Can you work these out from the model? Positions are in its coordinate system, mm. Face numbers are marked on the shaded views. Round coordinates to 2 decimals unless told otherwise and drop trailing zeros. Order: outer loops, then holes, each group sorted by start corner. A loop starts at its lowest first (then second) coordinate and runs counter-clockwise, first axis right, second up.
Q1. If we section it at B-B (y = 35): Please give me the cut outline in (x, z).
Q2. If I drill on line 1 (Z direction, x = 2, y = 7); line 2 (Z direction, x = 32, y = 17); line 3 (X direction, y = 4.5, z = -5), over which ranges is the centre line in solid material (lowest first)?
Q3. Will these pins go through, and if not, where does the flat tip stop? P1, Ø3, axis at x = 28.5, z = -0.5, coming from the +Y side; P2, Ø1.5, axis at y = 42, z = 2, coming from the -X side; P3, Ø3, axis at x = 75.5, y = 16, coming from the -Z side; P4, Ø1.1, axis at y = 8.5, z = 4, coming from the -X side.
Q4. If we section it at C-C (x = 2): Please give me the cut outline in (y, z), plus the area to 3 significant figures.
Q5. We'd pull the mould along Z, two halves only. Please class the marked faces 1, 2 and 3: pulls with the +Z half, pulls with the -Z half, needs draft (parallel to the pull), parting line crosses it, or undercut.
Q6. If we section it at A-A (z = -5): Please give me the cut outline in (x, y), plus the area to 3 significant figures.
Q7. If we section it at D-D (x = 46): Please give me the cut outline in (y, z).
from build123d import *

# Parameters (mm, degrees)
SKETCH1_R               = 5.501178274
BOSS_EXTRUDE1_DEPTH     = 5
SKETCH2_R               = 8
SKETCH2_R_2             = 5
BOSS_EXTRUDE2_DEPTH     = 70
CUT_EXTRUDE1_DEPTH      = 123.755855257
CUT_EXTRUDE1_DEPTH_BACK = 123.755855257
SKETCH3_W               = 17.823798536
SKETCH3_H               = 40


with BuildPart() as part:
    # Sketch1 → Boss-Extrude1 (new body)
    with BuildSketch(Plane.XY):
        Polygon((0, 0), (0, 15), (11.823798536, 15), (11.823798536, 55), (0, 55), (0, 70), (70.043570566, 70), (100, 47.532677925), (100, 22.467322075), (70.043570566, 0), align=None)
        with Locations((41.814977969, 55)):
            Circle(SKETCH1_R, mode=Mode.SUBTRACT)
        with Locations((41.814977969, 15)):
            Circle(SKETCH1_R, mode=Mode.SUBTRACT)
        with Locations((79.789963406, 35)):
            Circle(SKETCH1_R, mode=Mode.SUBTRACT)
    extrude(amount=BOSS_EXTRUDE1_DEPTH)

    # Sketch2 → Boss-Extrude2 (add)
    with BuildSketch(Plane(origin=(0, 0, 0), x_dir=(1, 0, 0), z_dir=(0, 1, 0))):
        with Locations(Location((2, 5, 0), (0, 0, 321.317812547))):
            Circle(SKETCH2_R)
        with Locations(Location((2, 5, 0), (0, 0, 270))):
            Circle(SKETCH2_R_2, mode=Mode.SUBTRACT)
    extrude(amount=BOSS_EXTRUDE2_DEPTH)

    # Sketch3 → Cut-Extrude1 (cut, two sides: drawn at the far end of the back side and taken through both)
    with BuildSketch(Plane.XY.offset(-CUT_EXTRUDE1_DEPTH_BACK)):
        with Locations((2.911899268, 35)):
            Rectangle(SKETCH3_W, SKETCH3_H)
    extrude(amount=CUT_EXTRUDE1_DEPTH + CUT_EXTRUDE1_DEPTH_BACK, mode=Mode.SUBTRACT)


solid = part.part
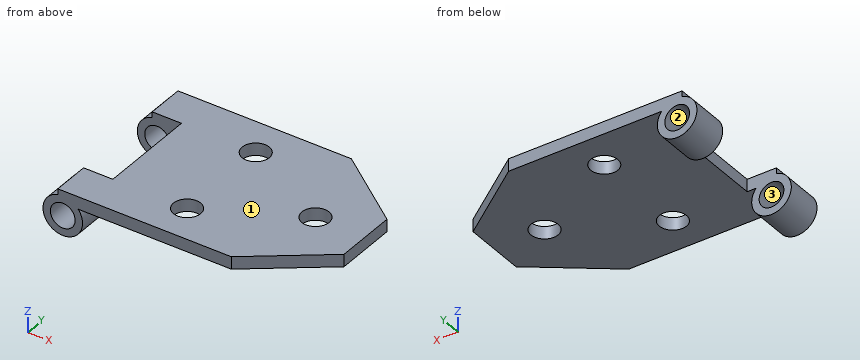
Solution:
1. outline: (11.82, 0) - (74.29, 0) - (74.29, 5) - (11.82, 5) - close; (85.29, 0) - (100, 0) - (100, 5) - (85.29, 5) - close
2. line 1: z = -13 to -10, 0 to 5
2. line 2: z = 0 to 5
2. line 3: x = -6 to -3, 7 to 10
3. P1: stops at y = 70
3. P2: stops at x = 11.82
3. P3: stops at z = 0
3. P4: stops at x = 0
4. outline: (0, -13) - (15, -13) - (15, -10) - (0, -10) - close; (0, 0) - (15, 0) - (15, 5) - (0, 5) - close; (55, -13) - (70, -13) - (70, -10) - (55, -10) - close; (55, 0) - (70, 0) - (70, 5) - (55, 5) - close
4. area: 240 mm2
5. face 1: pulls with the +Z half
5. face 2: undercut
5. face 3: undercut
6. outline: (-6, 0) - (-3, 0) - (-3, 15) - (-6, 15) - close; (-6, 55) - (-3, 55) - (-3, 70) - (-6, 70) - close; (7, 0) - (10, 0) - (10, 15) - (7, 15) - close; (7, 55) - (10, 55) - (10, 70) - (7, 70) - close
6. area: 180 mm2
7. outline: (0, 0) - (11.43, 0) - (11.43, 5) - (0, 5) - close; (18.57, 0) - (51.43, 0) - (51.43, 5) - (18.57, 5) - close; (58.57, 0) - (70, 0) - (70, 5) - (58.57, 5) - close
